Model file for the job. Use its own axes, mm. Coordinates: 2 decimals unless noted, no trailing zeros. Write each loop counter-clockwise with the first axis right and the second up, starting at its lowest first coordinate (ties: lowest second). Pieces come first, ordered by that corner, then holes. Notation, with made-up numbers: M -21,18 L 28,18 A20 cw 28,49 Z; hole C -25,52.5 d8. An arc over 180 degrees is marked long. One line per question, with ' | ' between items. Start each with the question number.
(1) Wall check: probe 1 along Y at (x, z) = (-0.2, 19); probe 2 along Y at (x, z) = (-0.3, 26); probe 3 along Y at (x, z) = (-0.1, 35.5). Give the ranges that are in metal, low to high.
(2) Cut at A-A (z = -20). Write the cut outline in (x, y), plus the area to 3 significant figures.
(3) Cut at D-D (z = -38). Write the cut outline in (x, y).
(4) Cut at C-C (z = 16.5). Write the cut outline in (x, y), plus the area to 3 significant figures.
(5) Two-plate mould, pull along Y, no slides. Class faces 1 (the face through (-0.246, 15.173, -23.611)), 2 (the face through (-0.25, 18.57, 20.71)), 3 (the face through (-0.25, -0.88, -44.57)): +Y half, -Y half, draft (parallel to the pull), parting line (faces both ways), or undercut.
(6) Cut at B-B (x = -0.4). Count the separate pieces of the cut face and the enclosed holes in it, plus the area to 3 significant figures.
from build123d import *

# Parameters (mm, degrees)
CROQUIS1_R        = 1.5
CROQUIS1_R_2      = 4
BRIDA_BASE1_DEPTH = 0.5


# Sheet-metal steps are written as plain solids
with BuildPart() as part:
    # Croquis1 → Brida base1 (new body)
    with BuildSketch(Plane(origin=(0, 0, 0), x_dir=(0, 0, -1), z_dir=(1, 0, 0))):
        with BuildLine():
            Line((-43.604767051, 5.805989848), (4.028698849, 5.805989848))
            Line((4.028698849, 5.805989848), (34.694125945, -5.355312836))
            ThreePointArc((34.694125945, -5.355312836), (44.627399867, -0.723351136), (39.995438167, 9.209922786))
            Line((39.995438167, 9.209922786), (6.76176705, 21.305989848))
            Line((6.76176705, 21.305989848), (-43.604767051, 21.305989848))
            ThreePointArc((-43.604767051, 21.305989848), (-51.354767051, 13.555989848), (-43.604767051, 5.805989848))
        make_face()
        with Locations((-19.604767051, 17.555989848)):
            Circle(CROQUIS1_R, mode=Mode.SUBTRACT)
        with Locations(Location((-19.604767051, 9.555989848, 0), (0, 0, 180))):
            Circle(CROQUIS1_R, mode=Mode.SUBTRACT)
        with Locations((-43.604767051, 13.555989848)):
            Circle(CROQUIS1_R, mode=Mode.SUBTRACT)
        with Locations((23.380149081, 11.2667268)):
            Circle(CROQUIS1_R, mode=Mode.SUBTRACT)
        with Locations(Location((20.643987934, 3.749185834, 0), (0, 0, 180))):
            Circle(CROQUIS1_R, mode=Mode.SUBTRACT)
        with Locations((-28.604767051, 13.555989848)):
            Circle(CROQUIS1_R_2, mode=Mode.SUBTRACT)
        with Locations((30.897690047, 8.530565653)):
            Circle(CROQUIS1_R, mode=Mode.SUBTRACT)
        with Locations(Location((28.161528901, 1.013024687, 0), (0, 0, 180))):
            Circle(CROQUIS1_R, mode=Mode.SUBTRACT)
        with Locations((-11.604767051, 17.555989848)):
            Circle(CROQUIS1_R, mode=Mode.SUBTRACT)
        with Locations(Location((-11.604767051, 9.555989848, 0), (0, 0, 180))):
            Circle(CROQUIS1_R, mode=Mode.SUBTRACT)
    extrude(amount=-BRIDA_BASE1_DEPTH)


solid = part.part
Filled in:
1) probe 1: 5.81 to 8.18, 10.93 to 16.18, 18.93 to 21.31 | probe 2: 5.81 to 10.52, 16.59 to 21.31 | probe 3: 5.81 to 21.31
2) outline: M -0.5,-0.01 L 0,-0.01 L 0,2.39 L -0.5,2.39 Z; M -0.5,5.1 L 0,5.1 L 0,16.49 L -0.5,16.49 Z | area: 6.89 mm²
3) outline: M -0.5,-5.79 L 0,-5.79 L 0,9.94 L -0.5,9.94 Z
4) outline: M -0.5,5.81 L 0,5.81 L 0,21.31 L -0.5,21.31 Z | area: 7.75 mm²
5) face 1: +Y half | face 2: undercut | face 3: parting line
6) separate pieces: 1 | enclosed holes: 10 | area: 1,360 mm²
